from build123d import *


with BuildPart() as part:
    # Sketch1 → Revolve1 (revolve)
    with BuildSketch(Plane.YZ, mode=Mode.PRIVATE) as revolve1_sk:
        Polygon((-28.5, 32.5), (-28.5, 5), (-12.1, 5), (-12.1, 10), (-20, 10), (-20, 25), (-23.5, 25), (-23.5, 37.5), (-25.5, 37.5), (-25.5, 38.5), (-27.5, 38.5), (-27.5, 37.5), (-29.5, 37.5), (-29.5, 38.5), (-31.5, 38.5), (-31.5, 37.5), (-33.5, 37.5), (-33.5, 38.5), (-35.5, 38.5), (-35.5, 37.5), (-37.5, 37.5), (-37.5, 38.5), (-39.5, 38.5), (-39.5, 37.5), (-63.5, 37.5), (-63.5, 5), (-132.334, 5), (-132.334, 0), (-60.5, 0), (-60.5, 32.5), align=None)
    revolve(revolve1_sk.sketch.rotate(Axis((0, 0, 1538.348894466), (0, 0, -1)), 270), axis=Axis((0, 0, 1538.348894466), (0, 0, -1)))


solid = part.part
The listing builds one solid part. Answer for the finished solid, in the listing's coordinates (mm). A direction names the side the tool comes from. Give positions to 0.01 mm unless a question says otherwise; leave off trailing zeros. Write each loop counter-clockwise with the first axis right and the second up, starting at its lowest first coordinate (ties: lowest second). Pieces come first, ordered by that corner, then holes.
1) A tool of negligible diameter and unlimited length cuts with its end or side. For faces 1 (the face through (-6.18, 27.82, 18.56)), 2 (the face through (11.541, -3.635, 7.535)), 3 (the face through (15.5, 29.7, 38)), from which of +Z, -Z, +X, -X, +Y, -Y can it reach the whole face along a straight path? Write none if from no direction.
2) Section B-B (x = 47) is taken. Write down the section's boundary in (y, z), and give its area (3 significant figures).
3) For a pull along X with two mould halves and no side action, classify faces 4 (the face through (-33, 14, 37.5)), 5 (the face through (-105.02, 80.52, 2.46)), 6 (the face through (-35, 14, 38.5)) as pulls with the +X half, pulls with the -X half, needs draft (parallel to the pull), parting line crosses it, or undercut.
4) Find the intervals of material crossed by L1, parallel to Y at x = 0, z = 15; L2, parallel to X at y = 5.5, z = 31; L3, parallel to X at y = 21.5, z = 9, in increasing order.
5) Section C-C (x = -107) is taken. Write down the section's boundary in (y, z), and give its area (3 significant figures).
6) Section A-A (y = 57) is taken. Write down the section's boundary in (x, z).
7) Given P1, Ø2, axis at x = 84.5, z = 5, coming from the +Y side; P2, Ø5, axis at y = 37.5, z = 34.5, coming from the +X side; P3, Ø3, axis at x = 92.5, y = 54.5, coming from the +Z side, each flat-ended and moving along its own axis, determine where each tip first touches the part or whether it passes through.
8) Section D-D (x = 97) is taken. Write down the section's boundary in (y, z).
Response:
1. face 1: -Z
1. face 2: +Z, -Z
1. face 3: +Z
2. outline: (-123.71, 0) - (-38.1, 0) - (-38.1, 32.5) - (38.1, 32.5) - (38.1, 0) - (123.71, 0) - (123.71, 5) - (42.7, 5) - (42.7, 37.5) - (-42.7, 37.5) - (-42.7, 5) - (-123.71, 5) - close
2. area: 1,540 mm2
3. face 4: undercut
3. face 5: parting line crosses it
3. face 6: needs draft
4. L1: y = -63.5 to -60.5, -28.5 to -20, 20 to 28.5, 60.5 to 63.5
4. L2: x = -63.26 to -60.25, -27.96 to -22.85, 22.85 to 27.96, 60.25 to 63.26
4. L3: x = -59.75 to -56.55, -18.71 to 18.71, 56.55 to 59.75
5. outline: (-77.87, 0) - (77.87, 0) - (77.87, 5) - (-77.87, 5) - close
5. area: 779 mm2
6. outline: (-119.43, 0) - (-20.28, 0) - (-20.28, 32.5) - (20.28, 32.5) - (20.28, 0) - (119.43, 0) - (119.43, 5) - (27.99, 5) - (27.99, 37.5) - (-27.99, 37.5) - (-27.99, 5) - (-119.43, 5) - close
7. P1: stops at y = 102.66
7. P2: stops at x = 52.98
7. P3: stops at z = 5
8. outline: (-90.02, 0) - (90.02, 0) - (90.02, 5) - (-90.02, 5) - close
